from build123d import *

# Parameters (mm, degrees)
F1_DEPTH = 25.4


with BuildPart() as f1:
    # F0 (on Top) → F1 (new body)
    with BuildSketch(Plane.XY):
        Polygon((-5.363799, -30.841844), (-5.661787, 18.326312), (-50.360113, 18.326312), (-50.360113, -30.841844), align=None)
        Polygon((5.359783, 18.39311), (-5.661787, 18.326312), (-5.363799, -30.841844), (5.658176, -30.841844), align=None)
        Polygon((51.552065, 18.326312), (5.359783, 18.39311), (5.658176, -30.841844), (51.850053, -30.841844), align=None)
    extrude(amount=F1_DEPTH)


solid = f1.part
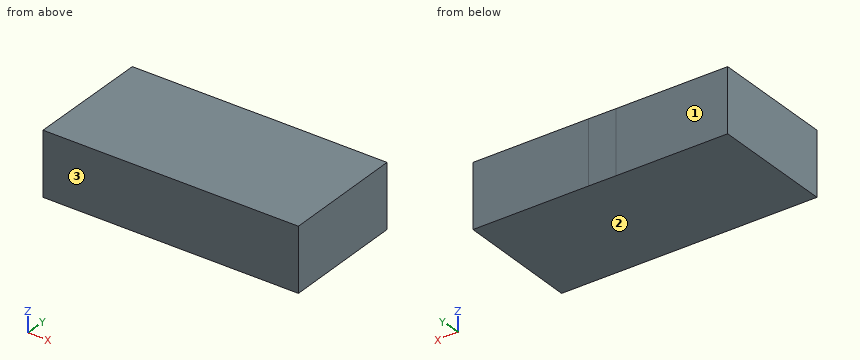
Here's how the part is built. I have some questions about the finished solid (model axes, mm). Face numbers are marked on the shaded views. Round coordinates to 2 decimals unless told otherwise and drop trailing zeros. Write each question's results on one line, items separated by ' | '.
(1) If I drill on L1, parallel to Y at x = 10.5, z = 11.5; L2, parallel to Y at x = 40, z = 17.5; L3, parallel to X at y = -10.5, z = 1, over which ranges is the centre line in solid material (lowest first)?
Worked answers:
L1: -30.84 to 18.39 | L2: -30.84 to 18.34 | L3: -50.36 to 51.73
(2) We'd pull the mould along Y, two halves only. Please class the marked faces 1, 2 and 3: released by +Y, released by -Y, zero draft, split by the parting line, or undercut.
Worked answers:
face 1: released by +Y | face 2: zero draft | face 3: released by -Y
(3) For P1, Ø12, axis at y = 5.5, z = 21, coming from the +X side; P2, Ø5, axis at x = -18.5, z = 13.5, coming from the +Y side, each with a flat end and sliding along its axis, tell me the tip position at first contact or that it passes through.
Worked answers:
P1: x = 51.67 | P2: y = 18.33
